Job drawing, mm, ordinate dimensions from the low corner. One solid piece. Give positions to 0.01 mm unless a question says otherwise; leave off trailing zeros. Loops run counter-clockwise (first coordinate to the right, second up) from the corner with the lowest first, then second, coordinate; pieces in that order, holes last.
Item 1: Drop flat-ended pins along their axis: P1, Ø3, axis at x = 6, y = 5, coming from the +Z side (1 decimal); P2, Ø4, axis at x = 3, z = 4, coming from the +Y side; P3, Ø4, axis at x = 5, z = 3.5, coming from the -Y side; P4, Ø1.5, axis at x = 3, z = 2.5, coming from the +Y side. Give the stop position or say it passes through.
Item 2: Saw through at B-B on y = 6. Give the cut face in (x, z), plus the area to 3 significant figures.
Item 3: Mould opens along Z. For the marked faces 1, 2 and 3 say: released by +Z, released by -Z, zero draft, split by the parting line, or undercut.
Item 4: Probe probe 1 along Z at (x, y) = (2.75, 4.5); probe 2 along X at (y, z) = (3.75, 3.25); probe 3 along Y at (x, z) = (4.5, 3.75). List the from-to ranges inside material, lowest first.
Item 5: Saw through at A-A on x = 1.5. Give the cut face in (y, z).
Item 6: Saw through at C-C on z = 2.25. Give the cut face in (x, y) (1 decimal).
Item 7: Saw through at D-D on x = 4.75. Give the cut face in (y, z).
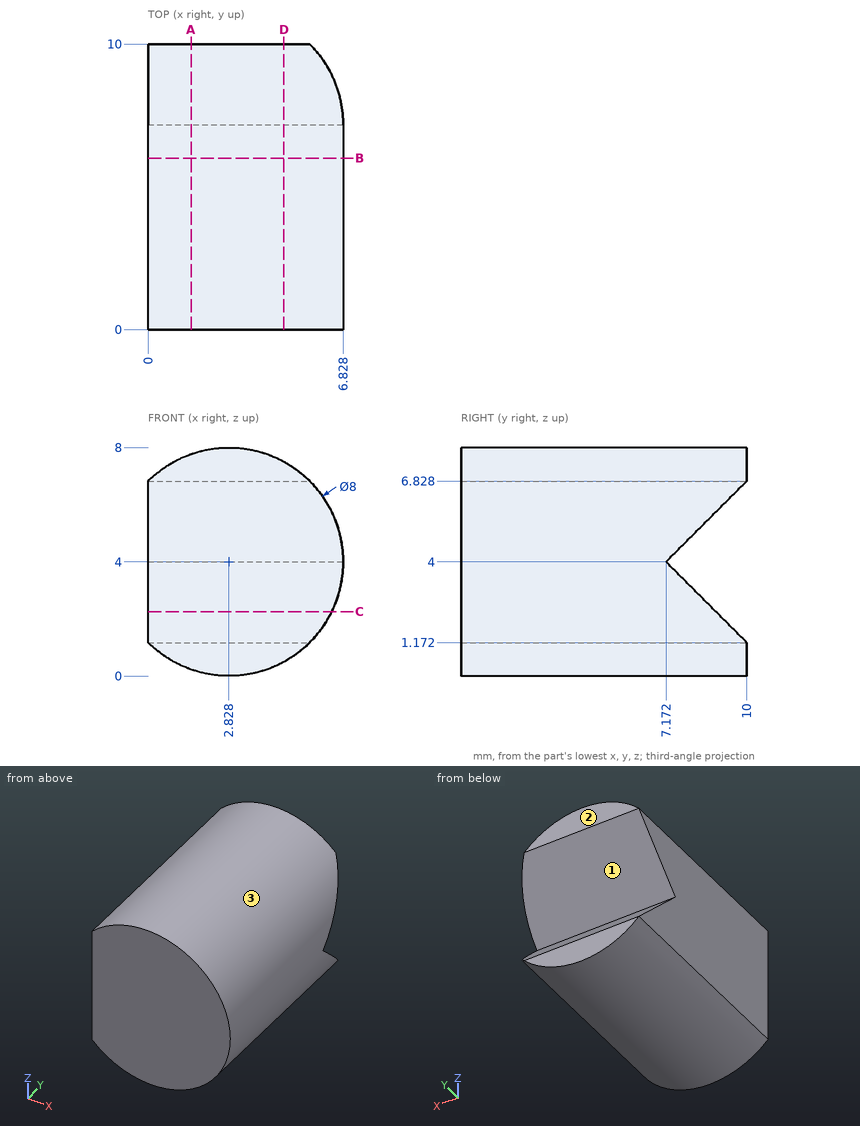
Results below:
1. P1: stops at z = 7.6
1. P2: stops at y = 9.17
1. P3: stops at y = 0
1. P4: stops at y = 9.42
2. outline: (0, 1.17) arc R4 ccw (long way) to (0, 6.83) - close
2. area: 45.7 mm2
3. face 1: undercut
3. face 2: zero draft
3. face 3: split by the parting line
4. probe 1: z = 0 to 8
4. probe 2: x = 0 to 6.76
4. probe 3: y = 0 to 7.42
5. outline: (0, 0.23) - (10, 0.23) - (10, 1.17) - (7.17, 4) - (10, 6.83) - (10, 7.77) - (0, 7.77) - close
6. outline: (0, 0) - (6.4, 0) - (6.4, 8.9) - (0, 8.9) - close
7. outline: (0, 0.49) - (10, 0.49) - (10, 1.17) - (7.17, 4) - (10, 6.83) - (10, 7.51) - (0, 7.51) - close
